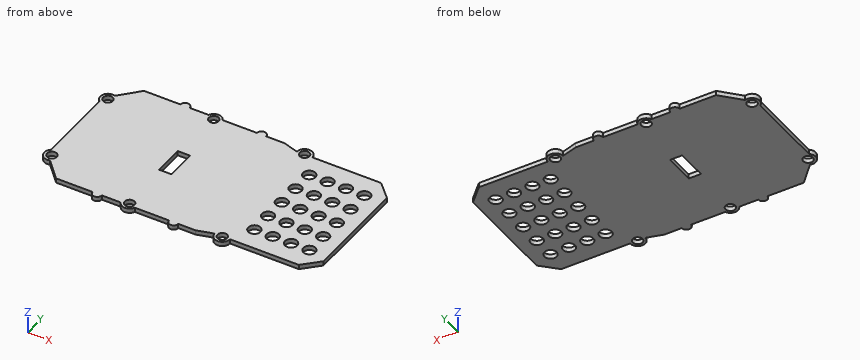
from build123d import *

# Parameters (mm, degrees)
F0_R     = 1.6
F0_W     = 4
F0_H     = 10
F0_R_2   = 2
F1_DEPTH = 1.5


# Not quite as in the source:
# - ends of sketch curves that miss each other by under 0.0002 mm in the source are joined


with BuildPart() as f1:
    # F0 (on Top) → F1 (new body)
    with BuildSketch(Plane.XY):
        with BuildLine():
            Line((25.1510733024, -23.3822189373), (30.8373828109, -23.3822189373))
            Line((30.8373828109, -23.3822189373), (36.1510733024, -21.8822189373))
            ThreePointArc((36.1510733024, -21.8822189373), (38.6560733124, -24.3822139373), (41.1510533024, -21.8722189373))
            Line((41.1510533024, -21.8722189373), (63.6510733024, -21.8722189373))
            Line((63.6510733024, -21.8722189373), (68.6510733024, -16.8822189373))
            Line((68.6510733024, -16.8822189373), (68.6510733024, 17.1177810627))
            Line((68.6510733024, 17.1177810627), (63.6510733024, 22.1277810627))
            Line((63.6510733024, 22.1277810627), (41.1510733024, 22.1277810627))
            ThreePointArc((41.1510733024, 22.1277810627), (38.6510733024, 24.6277810627), (36.1510733024, 22.1277810627))
            Line((36.1510733024, 22.1277810627), (31.0856380889, 23.6277810627))
            Line((31.0856380889, 23.6277810627), (25.1510399687, 23.6277810627))
            ThreePointArc((25.1510399687, 23.6277810627), (23.6460732747, 25.1177727292), (22.1510733024, 23.6177810627))
            Line((22.1510733024, 23.6177810627), (10.9423611499, 23.6177810627))
            ThreePointArc((10.9423611499, 23.6177810627), (8.6510733024, 25.1177810627), (6.359785455, 23.6177810627))
            Line((6.359785455, 23.6177810627), (0.1508824054, 23.6177810627))
            ThreePointArc((0.1508824054, 23.6177810627), (-1.3489266976, 25.0938508558), (-2.8487358005, 23.6177810627))
            Line((-2.8487358005, 23.6177810627), (-14.783491484, 23.6177810627))
            Line((-14.783491484, 23.6177810627), (-20.5213222757, 17.4701052144))
            ThreePointArc((-20.5213222757, 17.4701052144), (-23.5739450953, 16.2938104546), (-22.8489266976, 13.1037440347))
            Line((-22.8489266976, 13.1037440347), (-22.8489266976, -12.9160506452))
            ThreePointArc((-22.8489266976, -12.9160506452), (-23.5205541523, -16.0850132599), (-20.5005032054, -17.2566359677))
            Line((-20.5005032054, -17.2566359677), (-14.7737467559, -23.3822189373))
            Line((-14.7737467559, -23.3822189373), (-2.8489266976, -23.3822189373))
            ThreePointArc((-2.8489266976, -23.3822189373), (-1.3489266976, -24.8822189373), (0.1510733024, -23.3822189373))
            Line((0.1510733024, -23.3822189373), (6.359785455, -23.3822189373))
            ThreePointArc((6.359785455, -23.3822189373), (8.6510733024, -24.8822189373), (10.9423611499, -23.3822189373))
            Line((10.9423611499, -23.3822189373), (22.1510733024, -23.3822189373))
            ThreePointArc((22.1510733024, -23.3822189373), (23.6510729001, -24.8822181327), (25.1510733024, -23.3822189373))
        make_face()
        with Locations((-21.3217459931, -14.8953735334)):
            Circle(F0_R, mode=Mode.SUBTRACT)
        with Locations((8.6510733024, -22.3822189373)):
            Circle(F0_R, mode=Mode.SUBTRACT)
        with Locations((9.6388893649, 1.118e-07)):
            Rectangle(F0_W, F0_H, mode=Mode.SUBTRACT)
        with Locations((38.6510733024, -21.8822189373)):
            Circle(F0_R, mode=Mode.SUBTRACT)
        with Locations((44.6510733024, -14.5422189373)):
            Circle(F0_R_2, mode=Mode.SUBTRACT)
        with Locations((50.6510733024, -14.5422189373)):
            Circle(F0_R_2, mode=Mode.SUBTRACT)
        with Locations((56.6510733024, -14.5422189373)):
            Circle(F0_R_2, mode=Mode.SUBTRACT)
        with Locations((62.6510733024, -14.5422189373)):
            Circle(F0_R_2, mode=Mode.SUBTRACT)
        with Locations((44.6510733024, -7.2122189373)):
            Circle(F0_R_2, mode=Mode.SUBTRACT)
        with Locations((50.6510733024, -7.2122189373)):
            Circle(F0_R_2, mode=Mode.SUBTRACT)
        with Locations((56.6510733024, -7.2122189373)):
            Circle(F0_R_2, mode=Mode.SUBTRACT)
        with Locations((62.6510733024, -7.2122189373)):
            Circle(F0_R_2, mode=Mode.SUBTRACT)
        with Locations((-21.3678274943, 15.1177810627)):
            Circle(F0_R, mode=Mode.SUBTRACT)
        with Locations((8.6510733024, 22.6177810627)):
            Circle(F0_R, mode=Mode.SUBTRACT)
        with Locations((44.6510733024, 0.1277810627)):
            Circle(F0_R_2, mode=Mode.SUBTRACT)
        with Locations((44.6510733024, 7.4677810627)):
            Circle(F0_R_2, mode=Mode.SUBTRACT)
        with Locations((50.6510733024, 0.1277810627)):
            Circle(F0_R_2, mode=Mode.SUBTRACT)
        with Locations((56.6822756082, 0.1277810627)):
            Circle(F0_R_2, mode=Mode.SUBTRACT)
        with Locations((62.6510733024, 0.1277810627)):
            Circle(F0_R_2, mode=Mode.SUBTRACT)
        with Locations((50.6510733024, 7.4677810627)):
            Circle(F0_R_2, mode=Mode.SUBTRACT)
        with Locations((56.6510733024, 7.4677810627)):
            Circle(F0_R_2, mode=Mode.SUBTRACT)
        with Locations((62.6510733024, 7.4677810627)):
            Circle(F0_R_2, mode=Mode.SUBTRACT)
        with Locations((44.6510733024, 14.7977810627)):
            Circle(F0_R_2, mode=Mode.SUBTRACT)
        with Locations((38.6510733024, 22.1277810627)):
            Circle(F0_R, mode=Mode.SUBTRACT)
        with Locations((50.6510733024, 14.7977810627)):
            Circle(F0_R_2, mode=Mode.SUBTRACT)
        with Locations((56.6510733024, 14.7977810627)):
            Circle(F0_R_2, mode=Mode.SUBTRACT)
        with Locations((62.6510733024, 14.7977810627)):
            Circle(F0_R_2, mode=Mode.SUBTRACT)
    extrude(amount=F1_DEPTH)


solid = f1.part
Input: part model. Units: mm. Frame: model coordinates. Round coordinates to 2 decimals unless told otherwise and drop trailing zeros. Loops run counter-clockwise (first coordinate to the right, second up) from the corner with the lowest first, then second, coordinate; pieces in that order, holes last. Notation, with made-up numbers: (37, 31) -> (81, 31) arc R17 ccw to (81, 60) -> close; hole circle Ø5 at (59.25, -18). An arc over 180 degrees is marked (long way). Answer as a JSON object with one key per item and string values. Group by question number.
1) Section query D-D on z = 0.7. State how many separate pieces and enclosed holes the cut face has, plus the area to 3 significant figures.
2) Pin query (flat end, axial travel): pin 1 (12 mm diameter, centred on x = 25, y = -11.5, fed in from -Z); pin 2 (0.8 mm diameter, centred on x = -11, z = 1, fed in from +Y); pin 3 (0.8 mm diameter, centred on x = 1.5, z = 1, fed in from -Y); pin 4 (0.8 mm diameter, centred on y = 0.5, z = 0.5, fed in from -X). Return the tip coordinate at first contact, or that it passes through.
3) Section query B-B on x = 38.5. Output: boundary loops of the cut face in (y, z), plus the area to 3 significant figures.
4) Ray query, L1, parallel to X at y = 3, z = 1.15; L2, parallel to Y at x = 50, z = 0.7; L3, parallel to X at y = -1, z = 0.4. Return the intervals inside material, ascending.
5) Section query A-A on y = 8.5. Output: boundary loops of the cut face in (x, z), plus the area to 3 significant figures.
6) Section query C-C on x = 53.5. Output: boundary loops of the cut face in (y, z).
Reply:
{
 "1": {"separate pieces": "1", "enclosed holes": "27", "area": "3,820 mm2"},
 "2": {"pin 1": "stops at z = 0", "pin 2": "stops at y = 23.62", "pin 3": "stops at y = -23.38", "pin 4": "stops at x = -22.85"},
 "3": {"outline": "(-24.38, 0) -> (-23.48, 0) -> (-23.48, 1.5) -> (-24.38, 1.5) -> close; (-20.29, 0) -> (20.53, 0) -> (20.53, 1.5) -> (-20.29, 1.5) -> close; (23.72, 0) -> (24.62, 0) -> (24.62, 1.5) -> (23.72, 1.5) -> close", "area": "63.9 mm2"},
 "4": {"L1": "x = -22.85 to 7.64, 11.64 to 68.65", "L2": "y = -21.87 to -16.43, -12.65 to -9.1, -5.32 to -1.76, 2.02 to 5.58, 9.36 to 12.91, 16.69 to 22.13", "L3": "x = -22.85 to 7.64, 11.64 to 43, 46.3 to 49, 52.3 to 55.03, 58.33 to 61, 64.3 to 68.65"},
 "5": {"outline": "(-22.85, 0) -> (42.94, 0) -> (42.94, 1.5) -> (-22.85, 1.5) -> close; (46.36, 0) -> (48.94, 0) -> (48.94, 1.5) -> (46.36, 1.5) -> close; (52.36, 0) -> (54.94, 0) -> (54.94, 1.5) -> (52.36, 1.5) -> close; (58.36, 0) -> (60.94, 0) -> (60.94, 1.5) -> (58.36, 1.5) -> close; (64.36, 0) -> (68.65, 0) -> (68.65, 1.5) -> (64.36, 1.5) -> close", "area": "117 mm2"},
 "6": {"outline": "(-21.87, 0) -> (22.13, 0) -> (22.13, 1.5) -> (-21.87, 1.5) -> close"}
}
